The drawing under review shows one solid part. Ordinate dimensions are in mm from its lowest x, y, z. Give positions to 0.01 mm unless a question says otherwise; leave off trailing zeros. Loops run counter-clockwise (first coordinate to the right, second up) from the corner with the lowest first, then second, coordinate; pieces in that order, holes last. Notation, with made-up numbers: (39.5, 68) - (66.5, 68) arc R18 cw to (66.5, 97) - close; hole circle Ø1 at (31.5, 3.5). An arc over 180 degrees is marked (long way). Return JSON: item names as keys, results as strings. Group by question number.
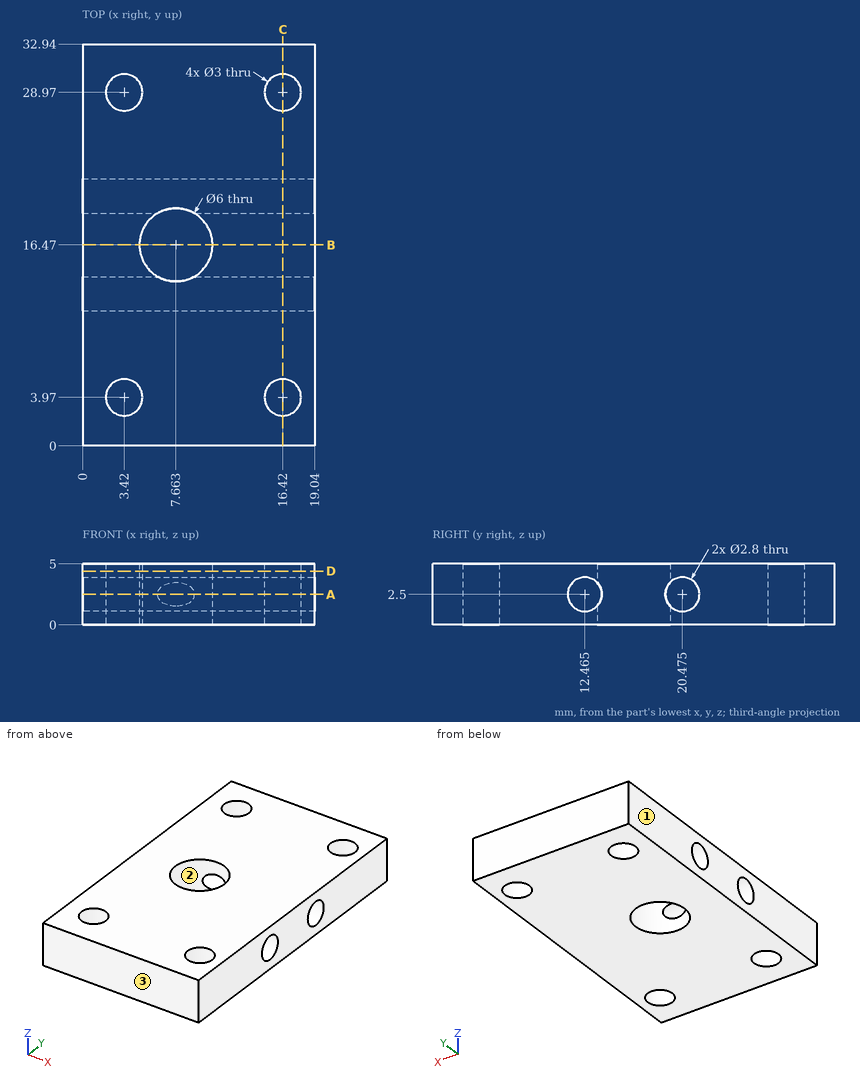
1) To check wall thickness, follow line 1 (Y direction, x = 3.5, z = 2.6); line 2 (Z direction, x = 10.5, y = 20.5); line 3 (Y direction, x = 16.42, z = 3.15) (1 decimal). State the ranges of each line that lie inside material, in increasing order.
2) For pin 1 Ø5.5 at (x, y) = (7.66, 16.47) entering from +Z; pin 2 Ø3.5 at (x, y) = (16.42, 28.97) entering from +Z, all flat-tipped, find the tip position at first contact; note any pin that passes through.
3) We need section C-C, the plane x = 16.42. Write out the cut boundary in (y, z) (1 decimal).
4) We need section D-D, the plane z = 4.4. Write out the cut boundary in (x, y).
5) We need section B-B, the plane y = 16.47. Write out the cut boundary in (x, z), plus the area to 3 significant figures.
6) Draft analysis for pull direction X (two halves, no side actions). For the marked faces 1, 2 and 3, state which applies: +X half, -X half, draft (parallel to the pull), parting line (faces both ways), or undercut.
7) We need section A-A, the plane z = 2.5. Write out the cut boundary in (x, y) (1 decimal).
Findings:
{
 "1": {"line 1": "y = 0 to 2.47, 5.47 to 11.07, 13.86 to 19.08, 21.87 to 27.47, 30.47 to 32.94", "line 2": "z = 0 to 1.1, 3.9 to 5", "line 3": "y = 0 to 2.5, 5.5 to 11.2, 13.7 to 19.2, 21.7 to 27.5, 30.5 to 32.9"},
 "2": {"pin 1": "passes through", "pin 2": "stops at z = 5"},
 "3": {"outline": "(0, 0) - (2.5, 0) - (2.5, 5) - (0, 5) - close; (5.5, 0) - (27.5, 0) - (27.5, 5) - (5.5, 5) - close; (30.5, 0) - (32.9, 0) - (32.9, 5) - (30.5, 5) - close; hole circle Ø2.8 at (12.5, 2.5); hole circle Ø2.8 at (20.5, 2.5)"},
 "4": {"outline": "(0, 0) - (19.04, 0) - (19.04, 32.94) - (0, 32.94) - close; hole circle Ø3 at (3.42, 3.97); hole circle Ø3 at (3.42, 28.97); hole circle Ø6 at (7.66, 16.47); hole circle Ø3 at (16.42, 3.97); hole circle Ø3 at (16.42, 28.97)"},
 "5": {"outline": "(0, 0) - (4.66, 0) - (4.66, 5) - (0, 5) - close; (10.66, 0) - (19.04, 0) - (19.04, 5) - (10.66, 5) - close", "area": "65.2 mm^2"},
 "6": {"face 1": "-X half", "face 2": "undercut", "face 3": "draft"},
 "7": {"outline": "(0, 0) - (19, 0) - (19, 11.1) - (0, 11.1) - close; (0, 13.9) - (6.2, 13.9) arc R3 cw to (6.2, 19.1) - (0, 19.1) - close; (0, 21.9) - (19, 21.9) - (19, 32.9) - (0, 32.9) - close; (9.2, 13.9) - (19, 13.9) - (19, 19.1) - (9.2, 19.1) arc R3 cw to start; hole circle Ø3 at (3.4, 4); hole circle Ø3 at (3.4, 29); hole circle Ø3 at (16.4, 4); hole circle Ø3 at (16.4, 29)"}
}
